Geometry: final body of the model. Coordinates: model frame, mm. A direction names the side the tool comes from. Give positions to 0.01 mm unless a question says otherwise; leave off trailing zeros. Order: outer loops, then holes, each group sorted by start corner. A loop starts at its lowest first (then second) coordinate and runs counter-clockwise, first axis right, second up. Notation, with made-up numbers: (27, 22) - (41, 22) arc R17 cw to (41, 45) - close; hole circle Ø8 at (-1.5, 81). An arc over 180 degrees is marked (long way). Use one line per item in the form item = value.
from build123d import *

# Parameters (mm, degrees)
SKETCH2_W           = 55
SKETCH2_H           = 70
BOSS_EXTRUDE1_DEPTH = 8
SKETCH3_R           = 25.5
CUT_EXTRUDE1_DEPTH  = 5
CUT_EXTRUDE3_DEPTH  = 125
SKETCH6_W           = 70
SKETCH6_H           = 1
CUT_EXTRUDE4_DEPTH  = 125


with BuildPart() as part:
    # Sketch2 → Boss-Extrude1 (new body)
    with BuildSketch(Plane(origin=(0, 0, 0), x_dir=(1, 0, 0), z_dir=(0, 1, 0))):
        Rectangle(SKETCH2_W, SKETCH2_H)
    extrude(amount=BOSS_EXTRUDE1_DEPTH)

    # Sketch3 → Cut-Extrude1 (cut)
    with BuildSketch(Plane(origin=(0, 8, 0), x_dir=(1, 0, 0), z_dir=(0, 1, 0))):
        with Locations(Location((0, 0, 0), (0, 0, 270))):
            Circle(SKETCH3_R)
    extrude(amount=-CUT_EXTRUDE1_DEPTH, mode=Mode.SUBTRACT)

    # Sketch4 → Cut-Extrude3 (cut)
    with BuildSketch(Plane(origin=(27.5, 0, 0), x_dir=(0, 0, -1), z_dir=(1, 0, 0))):
        with BuildLine():
            Line((-30.25, 0), (-30.25, 1.25))
            ThreePointArc((-30.25, 1.25), (-32.194543648, 2.055456352), (-33, 4))
            Line((-33, 4), (-33, 0))
            Line((-33, 0), (-30.25, 0))
        make_face()
        with BuildLine():
            ThreePointArc((-27.5, 4), (-28.305456352, 2.055456352), (-30.25, 1.25))
            Line((-30.25, 1.25), (-30.25, 0))
            Line((-30.25, 0), (-27.5, 0))
            Line((-27.5, 0), (-27.5, 4))
        make_face()
        with BuildLine():
            ThreePointArc((-27.5, 4), (-28.305456352, 5.944543648), (-30.25, 6.75))
            Line((-30.25, 6.75), (-30.25, 1.25))
            ThreePointArc((-30.25, 1.25), (-28.305456352, 2.055456352), (-27.5, 4))
        make_face()
        with BuildLine():
            Line((-30.25, 1.25), (-30.25, 6.75))
            ThreePointArc((-30.25, 6.75), (-32.194543648, 5.944543648), (-33, 4))
            ThreePointArc((-33, 4), (-32.194543648, 2.055456352), (-30.25, 1.25))
        make_face()
    cut_extrude3 = extrude(amount=-CUT_EXTRUDE3_DEPTH, mode=Mode.SUBTRACT)

    # Mirror1: Cut-Extrude3 across plane
    add(cut_extrude3.mirror(Plane.XY), mode=Mode.SUBTRACT)

    # Sketch6 → Cut-Extrude4 (cut)
    with BuildSketch(Plane(origin=(27.5, 0, 0), x_dir=(0, 0, -1), z_dir=(1, 0, 0))):
        with Locations((0, 0.5)):
            Rectangle(SKETCH6_W, SKETCH6_H)
    extrude(amount=-CUT_EXTRUDE4_DEPTH, mode=Mode.SUBTRACT)


solid = part.part
(1) Cut plane A-A on y = 5. Output: boundary loops of the cut face in (x, z), plus the area to 3 significant figures.
Computed values:
outline = (-27.5, -35) - (27.5, -35) - (27.5, -32.81) - (-27.5, -32.81) - close; (-27.5, -27.69) - (27.5, -27.69) - (27.5, 27.69) - (-27.5, 27.69) - close; (-27.5, 32.81) - (27.5, 32.81) - (27.5, 35) - (-27.5, 35) - close; hole circle Ø51 at (0, 0)
area = 1,240 mm²
(2) Cut plane B-B on x = 0. Output: boundary loops of the cut face in (y, z).
Computed values:
outline = (1, -35) - (8, -35) - (8, -25.5) - (3, -25.5) - (3, 25.5) - (8, 25.5) - (8, 35) - (1, 35) - (1, 33) - (4, 33) arc R2.75 cw to (4, 27.5) - (1, 27.5) - (1, -27.5) - (4, -27.5) arc R2.75 cw to (4, -33) - (1, -33) - close
(3) Pull-direction query (X, two-part tool) for faces 1 (the face through (-27.5, 4, 0)), 2 (the face through (0, 3, 0)), 3 (the face through (0, 2, -27.5)), 4 (the face through (27.5, 4, 0)); classes: released by +X, released by -X, zero draft, split by the parting line, or undercut.
Computed values:
face_1 = released by -X
face_2 = undercut
face_3 = zero draft
face_4 = released by +X
(4) Ray query, line 1 along Z through (x, y) = (-13, 2.75); line 2 along Z through (x, y) = (-5.5, 4.25); line 3 along Z through (x, y) = (-15.5, 6). Return the intervals inside material, ascending.
Computed values:
line_1 = -35 to -33, -27.5 to 27.5, 33 to 35
line_2 = -35 to -32.99, -27.51 to -24.9, 24.9 to 27.51, 32.99 to 35
line_3 = -35 to -32.14, -28.36 to -20.25, 20.25 to 28.36, 32.14 to 35
(5) Cut plane C-C on z = 0. Output: boundary loops of the cut face in (x, y).
Computed values:
outline = (-27.5, 1) - (27.5, 1) - (27.5, 8) - (25.5, 8) - (25.5, 3) - (-25.5, 3) - (-25.5, 8) - (-27.5, 8) - close
(6) Reachability of faces 5 (the face through (-24.9, 5.5, -5.5)), 6 (the face through (0, 2, 27.5)), 7 (the face through (-25, 8, 7)) from +Z, -Z, +X, -X, +Y, -Y: full face, straight path, thin tool, end or side. Return the list, or none.
Computed values:
face_5 = +Y
face_6 = +X, -X, -Y
face_7 = +Z, -Z, +X, -X, +Y
(7) Contact query for a flat-ended pin moving along its axis: pin 1 Ø5 at (x, z) = (16, 14.5) entering from +Y. Output: stop coordinate, or through.
Computed values:
pin_1 = 3
(8) Cut plane D-D on x = 22.5. Output: boundary loops of the cut face in (y, z), plus the area to 3 significant figures.
Computed values:
outline = (1, -35) - (8, -35) - (8, -12) - (3, -12) - (3, 12) - (8, 12) - (8, 35) - (1, 35) - (1, 33) - (4, 33) arc R2.75 cw to (4, 27.5) - (1, 27.5) - (1, -27.5) - (4, -27.5) arc R2.75 cw to (4, -33) - (1, -33) - close
area = 313 mm²
